Here's how the part is built. I have some questions about the finished solid (model axes, mm). Face numbers are marked on the shaded views. A direction names the side the tool comes from. Coordinates: 2 decimals unless noted, no trailing zeros.
Item 1: Please list where these lines run through material, in increasing order: line 1 (X direction, y = -7.25, z = 9.25); line 2 (Y direction, x = 20, z = 7); line 3 (X direction, y = 4.5, z = 7).
Item 2: I want a section at A-A (x = -8). Count the separate pieces of the cut face and the enclosed holes in it, and give its area (3 significant figures).
Item 3: For the marked faces 1, 2 and 3, which set-ups out of +Z, -Z, +X, -X, +Y, -Y let a thin tool reach every point of the face, with its end or its side?
Item 4: I'm going to push flat-ended pins straight in: P1, Ø0.7, axis at x = -33, z = 9, coming from the +Y side; P2, Ø2, axis at y = -6.5, z = 11.5, coming from the +X side; P3, Ø8, axis at x = -39.5, y = -11, coming from the -Z side; P4, Ø5, axis at y = 10.5, z = 10, coming from the +X side. Where does each tip first touch, or does it pass through?
Item 5: If we mould it in two halves opening along X, with no side actions, what happens to the marked faces 4, 5 and 6? For each: pulls with the +X half, pulls with the -X half, needs draft (parallel to the pull), parting line crosses it, or undercut.
from build123d import *

# Parameters (mm, degrees)
F0_W     = 1.390167144
F0_H     = 13.0257857824
F1_DEPTH = 12.7


with BuildPart() as f1:
    # F0 (on Top) → F1 (new body)
    with BuildSketch(Plane.XY):
        with BuildLine():
            Line((-43.1278555505, 8.1087965258), (-43.1278555505, 11.6189617885))
            ThreePointArc((-43.1278555505, 11.6189617885), (-63.6173153539, 0), (-43.1278555505, -11.6189617885))
            Line((-43.1278555505, -11.6189617885), (-43.1278555505, -8.1087965258))
            ThreePointArc((-43.1278555505, -8.1087965258), (-60.7580848758, 0), (-43.1278555505, 8.1087965258))
        make_face()
        Polygon((37.9903619809, 11.6189617885), (-43.1278555505, 11.6189617885), (-43.1278555505, 8.1087965258), (-43.1278555505, -8.1087965258), (-43.1278555505, -11.6189617885), (38.5659746826, -11.6189617885), align=None)
        with BuildLine():
            Line((-22.5185390528, -7.0921576955), (-26.2202943379, 2.1327664737))
            Line((-26.2202943379, 2.1327664737), (-24.7283423163, 2.1327664737))
            Line((-24.7283423163, 2.1327664737), (-22.7194302586, -3.0984405247))
            add(Edge.make_bspline(
                [(-22.7194302586, -3.0984405247), (-22.0605071037, -4.8903900802), (-21.899794139, -5.6859192551)],
                knots=[0, 0, 0, 1, 1, 1], degree=2))
            Line((-21.899794139, -5.6859192551), (-21.8328304038, -5.6859192551))
            add(Edge.make_bspline(
                [(-21.8328304038, -5.6859192551), (-21.7256884274, -5.2573513494), (-21.377477004, -4.223431277)],
                knots=[0, 0, 0, 1, 1, 1], degree=2))
            add(Edge.make_bspline(
                [(-21.377477004, -4.223431277), (-21.0292655807, -3.1895112047), (-19.1033885547, 2.1327664737)],
                knots=[0, 0, 0, 1, 1, 1], degree=2))
            Line((-19.1033885547, 2.1327664737), (-17.6141150825, 2.1327664737))
            Line((-17.6141150825, 2.1327664737), (-21.5569398145, -8.3135762266))
            add(Edge.make_bspline(
                [(-21.5569398145, -8.3135762266), (-22.1435421354, -9.8617777858), (-22.9256785632, -10.5113260178)],
                knots=[0, 0, 0, 1, 1, 1], degree=2))
            add(Edge.make_bspline(
                [(-22.9256785632, -10.5113260178), (-23.707814991, -11.1608742498), (-24.8461984904, -11.1608742498)],
                knots=[0, 0, 0, 1, 1, 1], degree=2))
            add(Edge.make_bspline(
                [(-24.8461984904, -11.1608742498), (-25.4836932501, -11.1608742498), (-26.1024381638, -11.0162325816)],
                knots=[0, 0, 0, 1, 1, 1], degree=2))
            Line((-26.1024381638, -11.0162325816), (-26.1024381638, -9.9046345763))
            add(Edge.make_bspline(
                [(-26.1024381638, -9.9046345763), (-25.6417276653, -10.0037409045), (-25.0738751903, -10.0037409045)],
                knots=[0, 0, 0, 1, 1, 1], degree=2))
            add(Edge.make_bspline(
                [(-25.0738751903, -10.0037409045), (-23.6408512558, -10.0037409045), (-23.0301419902, -8.3966112583)],
                knots=[0, 0, 0, 1, 1, 1], degree=2))
            Line((-23.0301419902, -8.3966112583), (-22.5185390528, -7.0921576955))
        make_face(mode=Mode.SUBTRACT)
        with BuildLine():
            Line((-32.4532788157, -2.3457681404), (-32.3863150805, -2.3457681404))
            add(Edge.make_bspline(
                [(-32.3863150805, -2.3457681404), (-32.0273894595, -1.834165203), (-31.2907883716, -1.0064934352)],
                knots=[0, 0, 0, 1, 1, 1], degree=2))
            Line((-31.2907883716, -1.0064934352), (-28.3283127238, 2.1327664737))
            Line((-28.3283127238, 2.1327664737), (-26.6783262871, 2.1327664737))
            Line((-26.6783262871, 2.1327664737), (-30.3961528686, -1.775237116))
            Line((-30.3961528686, -1.775237116), (-26.4185069943, -7.0412652567))
            Line((-26.4185069943, -7.0412652567), (-28.1006360239, -7.0412652567))
            Line((-28.1006360239, -7.0412652567), (-31.3416808104, -2.7046937614))
            Line((-31.3416808104, -2.7046937614), (-32.3863150805, -3.6100434621))
            Line((-32.3863150805, -3.6100434621), (-32.3863150805, -7.0412652567))
            Line((-32.3863150805, -7.0412652567), (-33.760410928, -7.0412652567))
            Line((-33.760410928, -7.0412652567), (-33.760410928, 5.9845205257))
            Line((-33.760410928, 5.9845205257), (-32.3863150805, 5.9845205257))
            Line((-32.3863150805, 5.9845205257), (-32.3863150805, -0.9234584035))
            add(Edge.make_bspline(
                [(-32.3863150805, -0.9234584035), (-32.3863150805, -1.3814903527), (-32.4532788157, -2.3457681404)],
                knots=[0, 0, 0, 1, 1, 1], degree=2))
        make_face(mode=Mode.SUBTRACT)
        with Locations((-15.4297580384, -0.5283723655)):
            Rectangle(F0_W, F0_H, mode=Mode.SUBTRACT)
        with BuildLine():
            add(Edge.make_bspline(
                [(-6.3267078674, -7.0707293002), (-6.982952473, -7.2100138696), (-7.9124091183, -7.2100138696)],
                knots=[0, 0, 0, 1, 1, 1], degree=2))
            add(Edge.make_bspline(
                [(-7.9124091183, -7.2100138696), (-9.9454281208, -7.2100138696), (-11.1226505866, -5.9698454926)],
                knots=[0, 0, 0, 1, 1, 1], degree=2))
            add(Edge.make_bspline(
                [(-11.1226505866, -5.9698454926), (-12.2998730524, -4.7296771156), (-12.2998730524, -2.5305880497)],
                knots=[0, 0, 0, 1, 1, 1], degree=2))
            add(Edge.make_bspline(
                [(-12.2998730524, -2.5305880497), (-12.2998730524, -0.3100705886), (-11.207024893, 0.995722249)],
                knots=[0, 0, 0, 1, 1, 1], degree=2))
            add(Edge.make_bspline(
                [(-11.207024893, 0.995722249), (-10.1141767336, 2.3015150865), (-8.2713347393, 2.3015150865)],
                knots=[0, 0, 0, 1, 1, 1], degree=2))
            add(Edge.make_bspline(
                [(-8.2713347393, 2.3015150865), (-6.5490274685, 2.3015150865), (-5.5445714396, 1.1671494112)],
                knots=[0, 0, 0, 1, 1, 1], degree=2))
            add(Edge.make_bspline(
                [(-5.5445714396, 1.1671494112), (-4.5401154107, 0.032783736), (-4.5401154107, -1.8261295548)],
                knots=[0, 0, 0, 1, 1, 1], degree=2))
            Line((-4.5401154107, -1.8261295548), (-4.5401154107, -2.7046937614))
            Line((-4.5401154107, -2.7046937614), (-10.8588134697, -2.7046937614))
            add(Edge.make_bspline(
                [(-10.8588134697, -2.7046937614), (-10.8159566791, -4.3198590558), (-10.0418558995, -5.1569057465)],
                knots=[0, 0, 0, 1, 1, 1], degree=2))
            add(Edge.make_bspline(
                [(-10.0418558995, -5.1569057465), (-9.26775512, -5.9939524373), (-7.8615166795, -5.9939524373)],
                knots=[0, 0, 0, 1, 1, 1], degree=2))
            add(Edge.make_bspline(
                [(-7.8615166795, -5.9939524373), (-6.3802788556, -5.9939524373), (-4.9338621741, -5.3752075235)],
                knots=[0, 0, 0, 1, 1, 1], degree=2))
            Line((-4.9338621741, -5.3752075235), (-4.9338621741, -6.6153759005))
            add(Edge.make_bspline(
                [(-4.9338621741, -6.6153759005), (-5.6704632619, -6.9314447309), (-6.3267078674, -7.0707293002)],
                knots=[0, 0, 0, 1, 1, 1], degree=2))
        make_face(mode=Mode.SUBTRACT)
    extrude(amount=F1_DEPTH)


solid = f1.part
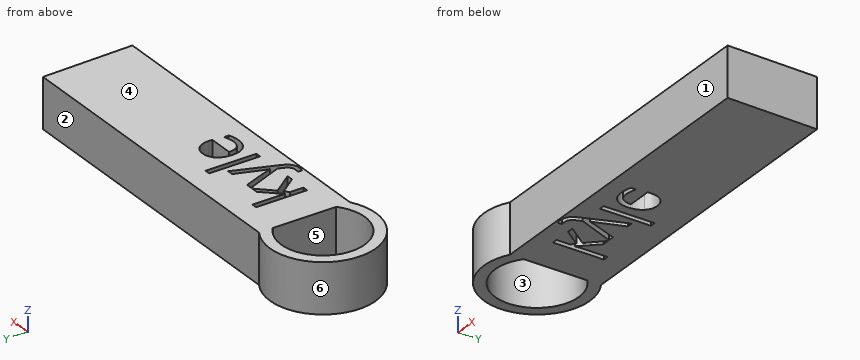
Answer:
1. line 1: x = -61.51 to -57.92, -43.13 to -22.58, -21.16 to 38.46
1. line 2: y = -11.62 to 11.62
1. line 3: x = -62.85 to -59.76, -43.13 to -33.76, -32.39 to -16.12, -14.73 to 38.17
2. separate pieces: 3
2. enclosed holes: 0
2. area: 216 mm2
3. face 1: +Z, -Z, +X, -Y
3. face 2: +Z, -Z, +X, +Y
3. face 3: +Z, -Z
4. P1: stops at y = 11.62
4. P2: stops at x = 38.46
4. P3: stops at z = 0
4. P4: stops at x = 38.08
5. face 4: needs draft
5. face 5: undercut
5. face 6: parting line crosses it
